from build123d import *

# Parameters (mm, degrees)
F0_W     = 12.7
F0_H     = 28.829
F0_W_2   = 6.35
F0_H_2   = 16.129
F0_W_3   = 5.715
F0_W_4   = 1.905
F1_DEPTH = 3.175
F2_DEPTH = 16.129
F3_R     = 3.2385
F4_DEPTH = 18.416
F5_R     = 1.27


with BuildPart() as f1:
    # F0 (on Top) → F1 (new body)
    with BuildSketch(Plane.XY):
        with Locations((0, 8.0645)):
            Rectangle(F0_W, F0_H)
        with Locations((0, 8.0645)):
            Rectangle(F0_W_2, F0_H_2, mode=Mode.SUBTRACT)
        with Locations((-9.2075, 8.0645)):
            Rectangle(F0_W_3, F0_H)
        with Locations((7.3025, 8.0645)):
            Rectangle(F0_W_4, F0_H)
    extrude(amount=F1_DEPTH)

    # F0 (on Top) → F2 (join)
    with BuildSketch(Plane.XY):
        with Locations((0, 8.0645)):
            Rectangle(F0_W, F0_H)
        with Locations((0, 8.0645)):
            Rectangle(F0_W_2, F0_H_2, mode=Mode.SUBTRACT)
    extrude(amount=F2_DEPTH)

    # F3 (on face) → F4 (cut, through all)
    with BuildSketch(Plane.YZ.offset(6.35)):
        with Locations((8.0645, 8.0645)):
            Circle(F3_R)
    extrude(amount=-F4_DEPTH, mode=Mode.SUBTRACT)

    # F5
    f5_edges = [f1.edges().sort_by_distance(p)[0] for p in [
        (3.175, 8.0645, 16.129),
        (-3.175, 8.0645, 16.129),
        (0, 0, 16.129),
        (0, 16.129, 16.129),
    ]]
    fillet(f5_edges, radius=F5_R)


solid = f1.part
CAD build for the part. Positions are in the model's coordinates, mm. A direction names the side the tool comes from. Coordinates: 2 decimals unless noted, no trailing zeros. Loops run counter-clockwise (first coordinate to the right, second up) from the corner with the lowest first, then second, coordinate; pieces in that order, holes last. Notation, with made-up numbers: (-2.75, 0) -> (40.25, 0) arc R5 ccw to (40.25, 9) -> close; hole circle Ø5 at (51, 88.5). An arc over 180 degrees is marked (long way). One line per item, written item: value.
1. Flat gauge pins, fed straight in: P1, Ø5, axis at y = 0, z = 8.5, coming from the +X side; P2, Ø1, axis at y = 0, z = 5, coming from the -X side; P3, Ø3, axis at x = -8, y = 6.5, coming from the +Z side (3 decimals); P4, Ø6, axis at y = 8.06, z = 8.06, coming from the -X side. Where does each tip first touch, or does it go through?
Answers:
P1: stops at x = 6.35
P2: stops at x = -6.35
P3: stops at z = 3.175
P4: passes through
2. Pull direction Y, two halves, no side cores. Call faces 1 (the face through (-12.065, 8, 2)), 2 (the face through (-2, 22.479, 8)), 3 (the face through (-3.56, 8.2, 15.77)): pulls with the +Y half, pulls with the -Y half, needs draft (parallel to the pull), parting line crosses it, or undercut.
Answers:
face 1: needs draft
face 2: pulls with the +Y half
face 3: undercut
3. Slice it at A-A on x = -2.75. Write the cut outline in (y, z), and give its area (3 significant figures).
Answers:
outline: (-6.35, 0) -> (0, 0) -> (0, 14.86) arc R1.27 ccw to (-1.27, 16.13) -> (-6.35, 16.13) -> close; (16.13, 0) -> (22.48, 0) -> (22.48, 16.13) -> (17.4, 16.13) arc R1.27 ccw to (16.13, 14.86) -> close
area: 204 mm^2
4. Slice it at D-D on z = 6.5. Write the cut outline in (x, y) (3 decimals), and give its area (3 significant figures).
Answers:
outline: (-6.35, -6.35) -> (6.35, -6.35) -> (6.35, 5.229) -> (3.175, 5.229) -> (3.175, 0) -> (-3.175, 0) -> (-3.175, 5.229) -> (-6.35, 5.229) -> close; (-6.35, 10.9) -> (-3.175, 10.9) -> (-3.175, 16.129) -> (3.175, 16.129) -> (3.175, 10.9) -> (6.35, 10.9) -> (6.35, 22.479) -> (-6.35, 22.479) -> close
area: 228 mm^2
5. Drill centre lines: line 1 (Y direction, x = -0.75, z = 3.75); line 2 (X direction, y = 8.25, z = 14.25) (3 decimals); line 3 (Z direction, x = -9.25, y = 15.5) (3 decimals). Where is each one in solid material? Low to high. Write a range as [from, to].
Answers:
line 1: y = [-6.35, 0], [16.13, 22.48]
line 2: x = [-6.35, -3.175], [3.175, 6.35]
line 3: z = [0, 3.175]
6. Which spindle directions (+Z, -Z, +X, -X, +Y, -Y) get a long thin tool onto all of the face, cutting with end or side? Do faces 4 (the face through (-6.35, 8, 12)), 5 (the face through (0.062, 16.511, 15.767)), 6 (the face through (0, 0, 7)). Say none if no direction does.
Answers:
face 4: +Z, -X, +Y, -Y
face 5: +Z
face 6: +Z, -Z
7. Slice it at B-B on y = 3.75. Write the cut outline in (x, z) (3 decimals).
Answers:
outline: (-12.065, 0) -> (-3.175, 0) -> (-3.175, 14.859) arc R1.27 ccw to (-4.445, 16.129) -> (-6.35, 16.129) -> (-6.35, 3.175) -> (-12.065, 3.175) -> close; (3.175, 0) -> (8.255, 0) -> (8.255, 3.175) -> (6.35, 3.175) -> (6.35, 16.129) -> (4.445, 16.129) arc R1.27 ccw to (3.175, 14.859) -> close
8. Slice it at C-C on z = 1.5. Write the cut outline in (x, y) (3 decimals).
Answers:
outline: (-12.065, -6.35) -> (8.255, -6.35) -> (8.255, 22.479) -> (-12.065, 22.479) -> close; hole (-3.175, 0) -> (3.175, 0) -> (3.175, 16.129) -> (-3.175, 16.129) -> close
